from build123d import *

# Parameters (mm, degrees)
SKETCH1_W           = 40
SKETCH1_H           = 3
BOSS_EXTRUDE1_DEPTH = 51.35
SKETCH2_W           = 3
SKETCH2_H           = 40
BOSS_EXTRUDE2_DEPTH = 10
FILLET1_R           = 3
SKETCH3_W           = 40
SKETCH3_H           = 2
BOSS_EXTRUDE3_DEPTH = 2
SKETCH4_W           = 30.35
SKETCH4_H           = 34
BOSS_EXTRUDE4_DEPTH = 14.04
SKETCH5_W           = 3
SKETCH5_H           = 29.82
BOSS_EXTRUDE5_DEPTH = 10
FILLET3_R           = 1.5
SKETCH6_R           = 2.19
CUT_EXTRUDE1_DEPTH  = 68.601394216
CUT_EXTRUDE2_REACH  = 82.595
SKETCH7_R           = 1.5
SKETCH8_W           = 30.35
SKETCH8_H           = 34
CUT_EXTRUDE3_DEPTH  = 3


with BuildPart() as part:
    # Sketch1 → Boss-Extrude1 (new body)
    with BuildSketch(Plane(origin=(0, 0, 0), x_dir=(0, 0, -1), z_dir=(1, 0, 0))):
        with Locations((20, 1.5)):
            Rectangle(SKETCH1_W, SKETCH1_H)
    extrude(amount=BOSS_EXTRUDE1_DEPTH)

    # Sketch2 → Boss-Extrude2 (add)
    with BuildSketch(Plane(origin=(0, 3, 0), x_dir=(1, 0, 0), z_dir=(0, 1, 0))):
        with Locations((49.85, 20)):
            Rectangle(SKETCH2_W, SKETCH2_H)
    extrude(amount=BOSS_EXTRUDE2_DEPTH)

    # Fillet1
    fillet1_edges = [part.edges().sort_by_distance(p)[0] for p in [
        (51.35, 13, -20),
    ]]
    fillet(fillet1_edges, radius=FILLET1_R - 0.0001)  # a hair under: the kernel refuses the full size

    # Sketch3 → Boss-Extrude3 (add)
    with BuildSketch(Plane.ZY.offset(-48.35)):
        with Locations((-20, 9)):
            Rectangle(SKETCH3_W, SKETCH3_H)
    extrude(amount=BOSS_EXTRUDE3_DEPTH)

    # Sketch4 → Boss-Extrude4 (add)
    with BuildSketch(Plane(origin=(0, 3, 0), x_dir=(1, 0, 0), z_dir=(0, 1, 0))):
        Polygon((0, 40), (3, 40), (38.35, 40), (38.35, 37), (38.35, 3), (38.35, 0), (3, 0), (0, 0), align=None)
        with Locations((20.175, 20)):
            Rectangle(SKETCH4_W, SKETCH4_H, mode=Mode.SUBTRACT)
    extrude(amount=BOSS_EXTRUDE4_DEPTH)

    # Sketch5 → Boss-Extrude5 (add)
    with BuildSketch(Plane.XY):
        with Locations((25.17, 21.95)):
            Rectangle(SKETCH5_W, SKETCH5_H)
    boss_extrude5 = extrude(amount=BOSS_EXTRUDE5_DEPTH)

    # Mirror2: Boss-Extrude5 across plane
    add(boss_extrude5.mirror(Plane(origin=(0, 0, -20), x_dir=(1, 0, 0), z_dir=(0, 0, -1))))

    # Fillet3
    fillet3_edges = [part.edges().sort_by_distance(p)[0] for p in [
        (23.67, 12.04, 0),
        (25.17, 7.04, 0),
        (23.67, 7.04, 5),
        (26.67, 12.04, 0),
        (26.67, 7.04, 5),
        (25.17, 7.04, 10),
        (23.67, 12.04, -40),
        (23.67, 7.04, -45),
        (25.17, 7.04, -50),
        (26.67, 7.04, -45),
        (26.67, 12.04, -40),
        (25.17, 7.04, -40),
    ]]
    fillet(fillet3_edges, radius=FILLET3_R - 0.0001)  # a hair under: the kernel refuses the full size

    # Sketch6 → Cut-Extrude1 (cut, through all)
    with BuildSketch(Plane(origin=(26.67, 0, 0), x_dir=(0, 0, -1), z_dir=(1, 0, 0))):
        with Locations((-5, 32.035)):
            Circle(SKETCH6_R)
        with Locations((-5, 21.865)):
            Circle(SKETCH6_R)
    cut_extrude1 = extrude(amount=-CUT_EXTRUDE1_DEPTH, mode=Mode.SUBTRACT)

    # Mirror3: Cut-Extrude1 across plane
    add(cut_extrude1.mirror(Plane(origin=(0, 0, -20), x_dir=(1, 0, 0), z_dir=(0, 0, -1))), mode=Mode.SUBTRACT)

    # Sketch7 → Cut-Extrude2 (cut, up to next)
    with BuildSketch(Plane.ZY, mode=Mode.PRIVATE) as cut_extrude2_sk1:
        with Locations((-10, 13.52)):
            Circle(SKETCH7_R)
    cut_extrude2_tool1 = extrude(cut_extrude2_sk1.sketch, amount=-CUT_EXTRUDE2_REACH, mode=Mode.PRIVATE) & part.part
    # Sketch7 → Cut-Extrude2 (cut, up to next)
    with BuildSketch(Plane.ZY, mode=Mode.PRIVATE) as cut_extrude2_sk2:
        with Locations((-10, 6.52)):
            Circle(SKETCH7_R)
    cut_extrude2_tool2 = extrude(cut_extrude2_sk2.sketch, amount=-CUT_EXTRUDE2_REACH, mode=Mode.PRIVATE) & part.part
    cut_extrude2_1 = cut_extrude2_tool1.solids().sort_by_distance((0, 13.52, -10))[0]
    add(cut_extrude2_1, mode=Mode.SUBTRACT)
    cut_extrude2_2 = cut_extrude2_tool2.solids().sort_by_distance((0, 6.52, -10))[0]
    add(cut_extrude2_2, mode=Mode.SUBTRACT)
    cut_extrude2 = cut_extrude2_1 + cut_extrude2_2  # Cut-Extrude2 as one shape, for the pattern or mirror that repeats it

    # Mirror4: Cut-Extrude2 across plane
    add(cut_extrude2.mirror(Plane(origin=(0, 0, -20), x_dir=(1, 0, 0), z_dir=(0, 0, -1))), mode=Mode.SUBTRACT)

    # Sketch8 → Cut-Extrude3 (cut)
    with BuildSketch(Plane(origin=(0, 3, 0), x_dir=(1, 0, 0), z_dir=(0, 1, 0))):
        with Locations((20.175, 20)):
            Rectangle(SKETCH8_W, SKETCH8_H)
    extrude(amount=-CUT_EXTRUDE3_DEPTH, mode=Mode.SUBTRACT)


solid = part.part
Verification items for the finished model (mm, model axes). A direction names the side the tool comes from. Round coordinates to 2 decimals unless told otherwise and drop trailing zeros. Loops run counter-clockwise (first coordinate to the right, second up) from the corner with the lowest first, then second, coordinate; pieces in that order, holes last. Notation, with made-up numbers: (47.5, 74) - (75.5, 74) arc R6 cw to (75.5, 84) - close; hole circle Ø4 at (57, 52.25). An arc over 180 degrees is marked (long way). Answer in a Markdown table with one row per item. Add a question column.
Q1. Gauge pin test, flat ends, axial feed: pin 1 (5 mm diameter, centred on y = 21, z = 6.5, fed in from -X); pin 2 (11 mm diameter, centred on y = 16.5, z = -46, fed in from -X); pin 3 (8 mm diameter, centred on x = 46, y = 14, fed in from +Z); pin 4 (11.5 mm diameter, centred on x = 20.5, z = -13.5, fed in from +Y). Record the tip position at first contact, or that the pin passes through.
Q2. Section check D-D on y = 29. Enter the section's corners in (x, z), plus the area to 3 significant figures.
Q3. Section check A-A on z = 5. State how many separate pieces and enclosed holes the cut face has, plus the area to 3 significant figures.
Q4. Section check B-B on x = 9. Enter the section's corners in (y, z).
Q5. Material ranges on line 1 (Y direction, x = 1.45, z = -30); line 2 (Y direction, x = 25.2, z = -45) (3 decimals); line 3 (Z direction, x = 9.5, y = 10), recorded low to high.
Q6. Release check for a two-part mould opening along Y. For faces 1 (the face through (25.191, 29.897, -45.475)), 2 (the face through (47, 10, -20)), 3 (the face through (26.24, 7.49, 5.81)) record: pulls with the +Y half, pulls with the -Y half, needs draft (parallel to the pull), parting line crosses it, or undercut.
Q7. Tool access check on faces 4 (the face through (2.46, 6.59, -28.5)), 5 (the face through (25, 27, 0)), 6 (the face through (38.35, 10, -20)). Record the directions out of +Z, -Z, +X, -X, +Y, -Y that give a thin tool (end or side, any length) a straight path to the whole face; none if there is none.
Found:
| question | item | result |
|---|---|---|
| 1 | pin 1 | stops at x = 23.67 |
| 1 | pin 2 | stops at x = 23.29 |
| 1 | pin 3 | stops at z = 0 |
| 1 | pin 4 | passes through |
| 2 | outline | (23.67, -50) - (26.67, -50) - (26.67, -40) - (23.67, -40) - close; (23.67, 0) - (26.67, 0) - (26.67, 10) - (23.67, 10) - close |
| 2 | area | 60.0 mm² |
| 3 | separate pieces | 3 |
| 3 | enclosed holes | 0 |
| 3 | area | 62.2 mm² |
| 4 | outline | (0, -40) - (17.04, -40) - (17.04, -37) - (0, -37) - close; (0, -3) - (17.04, -3) - (17.04, 0) - (0, 0) - close |
| 5 | line 1 | y = 0 to 5.02, 8.02 to 12.02, 15.02 to 17.04 |
| 5 | line 2 | y = 7.04 to 19.675, 24.055 to 29.845, 34.225 to 36.86 |
| 5 | line 3 | z = -40 to -37, -3 to 0 |
| 6 | face 1 | undercut |
| 6 | face 2 | pulls with the +Y half |
| 6 | face 3 | pulls with the -Y half |
| 7 | face 4 | -X |
| 7 | face 5 | +X, -X, +Y |
| 7 | face 6 | +Z, -Z, +Y |
